```python
from build123d import *

# Parameters (mm, degrees)
SKETCH1_R           = 1
BOSS_EXTRUDE1_DEPTH = 33.615
CUT_EXTRUDE1_DEPTH  = 39.782573705
SKETCH3_W           = 37.23
SKETCH3_H           = 14
CUT_EXTRUDE3_DEPTH  = 10


with BuildPart() as part:
    # Sketch1 → Boss-Extrude1 (new body)
    with BuildSketch(Plane(origin=(0, 0, 0), x_dir=(0, 0, -1), z_dir=(1, 0, 0))):
        with BuildLine():
            ThreePointArc((0, 15.7), (1.5, 19.022875656), (3, 15.7))
            Line((3, 15.7), (3, 0))
            Line((3, 0), (0, 0))
            Line((0, 0), (0, 15.7))
        make_face()
        with Locations((1.5, 17.022875656)):
            Circle(SKETCH1_R, mode=Mode.SUBTRACT)
    boss_extrude1 = extrude(amount=BOSS_EXTRUDE1_DEPTH)

    # Sketch2 → Cut-Extrude1 (cut, through all)
    with BuildSketch(Plane(origin=(0, 0, -3), x_dir=(-1, 0, 0), z_dir=(0, 0, -1))):
        with BuildLine():
            Line((-1.4, 13.1), (-1.4, 2.6))
            ThreePointArc((-1.4, 2.6), (-3, 1), (-4.6, 2.6))
            Line((-4.6, 2.6), (-4.6, 13.1))
            ThreePointArc((-4.6, 13.1), (-3, 14.7), (-1.4, 13.1))
        make_face()
    cut_extrude1 = extrude(amount=-CUT_EXTRUDE1_DEPTH, mode=Mode.SUBTRACT)

    # Mirror1: Boss-Extrude1, Cut-Extrude1 across plane
    add(boss_extrude1.mirror(Plane(origin=(33.615, 0, 0), x_dir=(0, 0, 1), z_dir=(1, 0, 0))))
    add(cut_extrude1.mirror(Plane(origin=(33.615, 0, 0), x_dir=(0, 0, 1), z_dir=(1, 0, 0))), mode=Mode.SUBTRACT)

    # Sketch3 → Cut-Extrude3 (cut)
    with BuildSketch(Plane(origin=(0, 0, -3), x_dir=(-1, 0, 0), z_dir=(0, 0, -1))):
        with Locations((-33.615, 7)):
            Rectangle(SKETCH3_W, SKETCH3_H)
    extrude(amount=-CUT_EXTRUDE3_DEPTH, mode=Mode.SUBTRACT)


solid = part.part
```
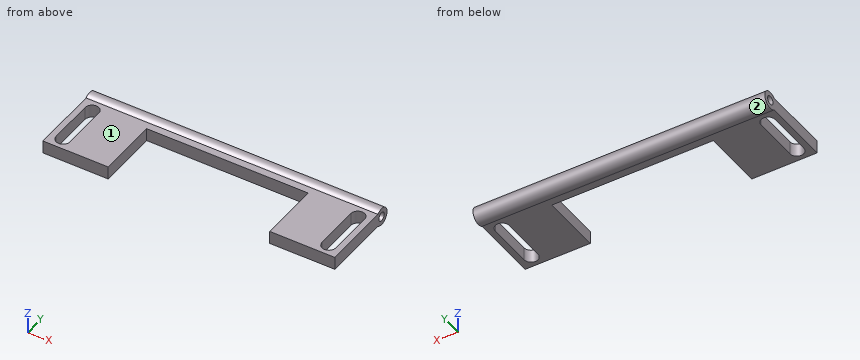
The model under review builds one solid part; all positions refer to its coordinate system, in mm. Face numbers are marked on the shaded views. Give positions to 0.01 mm unless a question says otherwise; leave off trailing zeros. Write each loop counter-clockwise with the first axis right and the second up, starting at its lowest first coordinate (ties: lowest second). Pieces come first, ordered by that corner, then holes. Notation, with made-up numbers: (0.5, 60) -> (8.5, 60) arc R15 ccw to (8.5, 64) -> close; hole circle Ø11 at (87.5, 79). An arc over 180 degrees is marked (long way). Put each result on its own line as item: value.
(1) We need section C-C, the plane x = 64.23. Give the boundary of the cut face in (y, z), and give its area (3 significant figures).
Results are:
outline: (0, -3) -> (1, -3) -> (1, 0) -> (0, 0) -> close; (14.7, -3) -> (15.7, -3) arc R2 ccw (long way) to (15.7, 0) -> (14.7, 0) -> close; hole circle Ø2 at (17.02, -1.5)
area: 14.0 mm²
(2) The part is to be moulded in two halves that separate along Y. For the marked faces 1 and 2, say which applies: pulls with the +Y half, pulls with the -Y half, needs draft (parallel to the pull), parting line crosses it, or undercut.
Results are:
face 1: needs draft
face 2: parting line crosses it
(3) To check wall thickness, follow probe 1 along X at (y, z) = (7.75, -1.75); probe 2 along Y at (x, z) = (17, -1.35); probe 3 along Y at (x, z) = (58, -1.4). State the ranges of each line that lie inside material, in increasing order. Write a range as from..to.
Results are:
probe 1: 0..1.4, 4.6..15, 52.23..62.63, 65.83..67.23
probe 2: 14..16.03, 18.01..19.02
probe 3: 0..16.03, 18.02..19.02
(4) We need section A-A, the plane z = -1.5. Give the boundary of the cut face in (x, y).
Results are:
outline: (0, 0) -> (15, 0) -> (15, 14) -> (52.23, 14) -> (52.23, 0) -> (67.23, 0) -> (67.23, 16.02) -> (0, 16.02) -> close; (0, 18.02) -> (67.23, 18.02) -> (67.23, 19.02) -> (0, 19.02) -> close; hole (1.4, 2.6) arc R1.6 ccw to (4.6, 2.6) -> (4.6, 13.1) arc R1.6 ccw to (1.4, 13.1) -> close; hole (62.63, 2.6) arc R1.6 ccw to (65.83, 2.6) -> (65.83, 13.1) arc R1.6 ccw to (62.63, 13.1) -> close
(5) We need section B-B, the plane y = 4.75. Give the boundary of the cut face in (x, z).
Results are:
outline: (0, -3) -> (1.4, -3) -> (1.4, 0) -> (0, 0) -> close; (4.6, -3) -> (15, -3) -> (15, 0) -> (4.6, 0) -> close; (52.23, -3) -> (62.63, -3) -> (62.63, 0) -> (52.23, 0) -> close; (65.83, -3) -> (67.23, -3) -> (67.23, 0) -> (65.83, 0) -> close
(6) For pin 1 Ø5 at (x, y) = (17.5, 16) entering from -Z; pin 2 Ø3 at (x, y) = (10, 9.5) entering from +Z; pin 3 Ø4 at (x, y) = (44, 13) entering from -Z, all flat-tipped, find the tip position at first contact; note any pin that passes through.
Results are:
pin 1: z = -3.5
pin 2: z = 0
pin 3: z = -3
(7) We need section D-D, the plane x = 7.5. Give the boundary of the cut face in (y, z), and give its area (3 significant figures).
Results are:
outline: (0, -3) -> (15.7, -3) arc R2 ccw (long way) to (15.7, 0) -> (0, 0) -> close; hole circle Ø2 at (17.02, -1.5)
area: 55.1 mm²
